For this review, take the finished solid that the model builds, in its own axes (mm). A direction names the side the tool comes from. Round coordinates to 2 decimals unless told otherwise and drop trailing zeros. Loops run counter-clockwise (first coordinate to the right, second up) from the corner with the lowest first, then second, coordinate; pieces in that order, holes last. Notation, with made-up numbers: (-12.75, -13.75) -> (22.25, -13.75) arc R25 ccw to (22.25, 22.25) -> close; hole circle Ø8 at (1.25, 3). An arc over 180 degrees is marked (long way). Use one line per item in the form item = value. Start each with the question number.
from build123d import *

# Parameters (mm, degrees)
F0_W     = 25.4
F0_H     = 76.2
F0_R     = 1.328071913
F1_DEPTH = 12.7
F2_T     = 2.54


# Not quite as in the source:
# - a shell that OpenCascade refuses in one call is made with other operations: the cavity is built on its own and cut out


with BuildPart() as f1:
    # F0 (on Front) → F1 (new body)
    with BuildSketch(Plane.XZ):
        Rectangle(F0_W, F0_H)
        with Locations((-11.0691860318, -36.4708118141)):
            Circle(F0_R, mode=Mode.SUBTRACT)
        with Locations((11.0691860318, -36.4708118141)):
            Circle(F0_R, mode=Mode.SUBTRACT)
        with Locations((-11.0691860318, 36.4708118141)):
            Circle(F0_R, mode=Mode.SUBTRACT)
        with Locations((11.0691860318, 36.4708118141)):
            Circle(F0_R, mode=Mode.SUBTRACT)
    extrude(amount=F1_DEPTH)

    # F2: shell of thickness 2.54, made by hand


with BuildPart() as f2_core1:
    # F2_t2: copy of F1
    add(f1.part)

    # the walls: a layer under each face that stays
    f2_faces = [f2_core1.faces().sort_by_distance(p)[0] for p in [
        (12.7, -6.35, 0),
        (-12.7, -6.35, 0),
        (0, -6.35, -38.1),
        (-12.3972579448, -6.35, -36.4708118141),
        (9.7411141188, -6.35, -36.4708118141),
        (-12.3972579448, -6.35, 36.4708118141),
        (9.7411141188, -6.35, 36.4708118141),
        (0, 0, 0),
        (0, -12.7, 0),
    ]]
    thicken(f2_faces, amount=-F2_T, mode=Mode.SUBTRACT)


with BuildPart() as f1_1:
    add(f1.part)

    # what is left inside the walls is the cavity
    f2_cavity = [f2_core1.part.solids().sort_by_distance(p)[0] for p in [
        (0, -2.5654, -11.006667),
    ]]
    add(f2_cavity, mode=Mode.SUBTRACT)


solid = f1_1.part
Item 1: For P1, Ø2.5, axis at x = 3, y = -6.5, coming from the +Z side, flat-tipped, find the tip position at first contact; note if it passes through.
Item 2: Take a section at C-C on y = -4. Give the boundary of the cut face in (x, z), plus the area to 3 significant figures.
Item 3: Machinability: for faces 1 (the flat face through (-12.7, -6, -1)), 2 (the cylindrical face through (8.36, -6.3, -33.71)), which of the approach directions +Z, -Z, +X, -X, +Y, -Y give a long, thin tool a straight path to every point of the face, cutting with its end or side? Answer none if there is none.
Item 4: Wall thickness on line 1 (Y direction, x = 3.25, z = -16); line 2 (X direction, y = -8.25, z = 18); line 3 (X direction, y = -6.75, z = -34.5): over which ranges is each line inside the solid? List them lowest first.
Item 5: Take a section at B-B on x = -6.25. Give the boundary of the cut face in (y, z), plus the area to 3 significant figures.
Item 6: Take a section at A-A on z = -12. Give the boundary of the cut face in (x, y).
Item 7: Take a section at D-D on x = 11.25. Give the boundary of the cut face in (y, z), plus the area to 3 significant figures.
Item 8: Draft analysis for pull direction X (two halves, no side actions). For faces 3 (the cylindrical face through (-8.31, -6.3, -33.76)), 4 (the flat face through (12.7, -6, -1)), 5 (the flat face through (0, -12.7, 1)), state which applies: +X half, -X half, draft (parallel to the pull), parting line (faces both ways), or undercut.
Results:
q1.P1 = -35.56
q2.outline = (-12.7, -38.1) -> (12.7, -38.1) -> (12.7, 38.1) -> (7.56, 38.1) arc R3.87 ccw to (10.16, 32.71) -> (10.16, -32.71) arc R3.87 ccw to (7.31, -35.56) -> (-7.31, -35.56) arc R3.87 ccw to (-10.16, -32.71) -> (-10.16, 32.71) arc R3.87 ccw to (-7.56, 38.1) -> (-12.7, 38.1) -> close; hole circle Ø2.66 at (-11.07, -36.47); hole circle Ø2.66 at (-11.07, 36.47); hole circle Ø2.66 at (11.07, -36.47); hole circle Ø2.66 at (11.07, 36.47)
q2.area = 454 mm2
q3.face_1 = +Z, -Z, -X, +Y, -Y
q3.face_2 = none
q4.line_1 = -12.7 to -10.16, -2.54 to 0
q4.line_2 = -12.7 to -10.16, 10.16 to 12.7
q4.line_3 = -12.7 to -7.74, 7.74 to 12.7
q5.outline = (-12.7, -38.1) -> (0, -38.1) -> (0, 38.1) -> (-2.54, 38.1) -> (-2.54, -35.56) -> (-10.16, -35.56) -> (-10.16, 38.1) -> (-12.7, 38.1) -> close
q5.area = 406 mm2
q6.outline = (-12.7, -12.7) -> (12.7, -12.7) -> (12.7, 0) -> (-12.7, 0) -> close; hole (-10.16, -10.16) -> (10.16, -10.16) -> (10.16, -2.54) -> (-10.16, -2.54) -> close
q7.outline = (-12.7, -38.1) -> (0, -38.1) -> (0, -37.79) -> (-12.7, -37.79) -> close; (-12.7, -35.16) -> (0, -35.16) -> (0, 35.16) -> (-12.7, 35.16) -> close; (-12.7, 37.79) -> (0, 37.79) -> (0, 38.1) -> (-12.7, 38.1) -> close
q7.area = 901 mm2
q8.face_3 = undercut
q8.face_4 = +X half
q8.face_5 = draft
